The listing builds one solid part. Answer for the finished solid, in the listing's coordinates (mm). Round coordinates to 2 decimals unless told otherwise and drop trailing zeros. Loops run counter-clockwise (first coordinate to the right, second up) from the corner with the lowest first, then second, coordinate; pieces in that order, holes last. Notation, with made-up numbers: M 60.5,0 L 74.5,0 A21 cw 74.5,21 Z; hole C -18,-33 d6. An arc over 180 degrees is marked long. Put each result on its own line as item: value. Start each with the question number.
(1) Flat-ended cylindrical pins translate along their axes: P1, Ø3, axis at x = 0, y = 0, coming from the +Z side; P2, Ø1, axis at x = -2.5, z = -8.5, coming from the -Y side. Find the tip coordinate at first contact, or state that the pin passes through.
(2) Section A-A, the plane z = 9.5 is taken. Determine the outline of the cut face in (x, y), then the cut area to 3 significant figures.
(3) Straight lines are drawn through the part: line 1 (Y direction, x = 0, z = 18.5); line 2 (X direction, y = 1.25, z = -17); line 3 (Z direction, x = -1.25, y = 1.5). For each, find the intervals that lie inside material, in ascending order.
(4) Section B-B, the plane x = 2.5 is taken. Determine the outline of the cut face in (y, z).
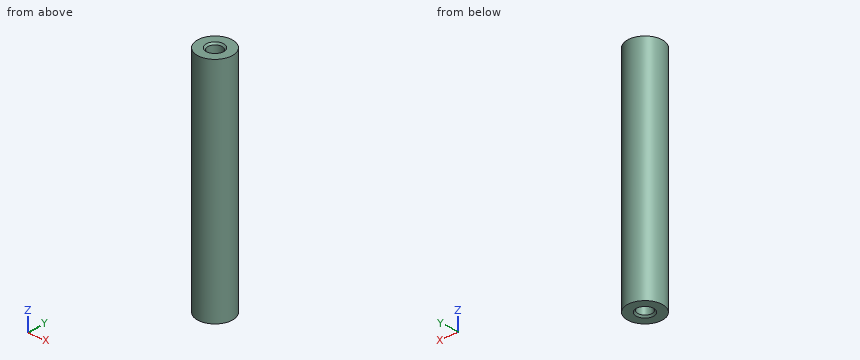
Autodesk Inventor part; units mm, degrees
ref_plane "YZ Plane" through (0, 0, 0) normal (1, 0, 0) x (0, 1, 0)
ref_plane "XZ Plane" through (0, 0, 0) normal (0, 1, 0) x (-1, 0, 0)
ref_plane "XY Plane" through (0, 0, 0) normal (0, 0, 1) x (1, 0, 0)
sketch "Sketch1" plane through (0, 0, 0) normal (0, 0, 1) x (1, 0, 0)
  circle A0 centre (0, 0) radius 4
  dimension "d0" = 8
extrude "Extrusion1" add sketch "Sketch1" along normal mid plane 52
sketch "Sketch2" plane through (0, 0, 26) normal (0, 0, 1) x (1, 0, 0)
  point P0 (0, 0)
  point P1 (0, 0)
hole "Hole1" at (0, 0, 26) direction (0, 0, -1) diameter 3.242 depth 11.8 tip angle 118 countersink diameter 4 countersink angle 90
mirror "Mirror1" about plane through (0, 0, 0) normal (0, 0, 1) of "Hole1"
properties part number "vul as platen"
Recorded:
1. P1: stops at z = 14.13
1. P2: stops at y = -3.46
2. outline: C 0,0 d8
2. area: 50.3 mm²
3. line 1: y = -4 to -1.62, 1.62 to 4
3. line 2: x = -3.8 to -1.03, 1.03 to 3.8
3. line 3: z = -25.95 to 25.95
4. outline: M -3.12,-26 L 3.12,-26 L 3.12,26 L -3.12,26 Z
